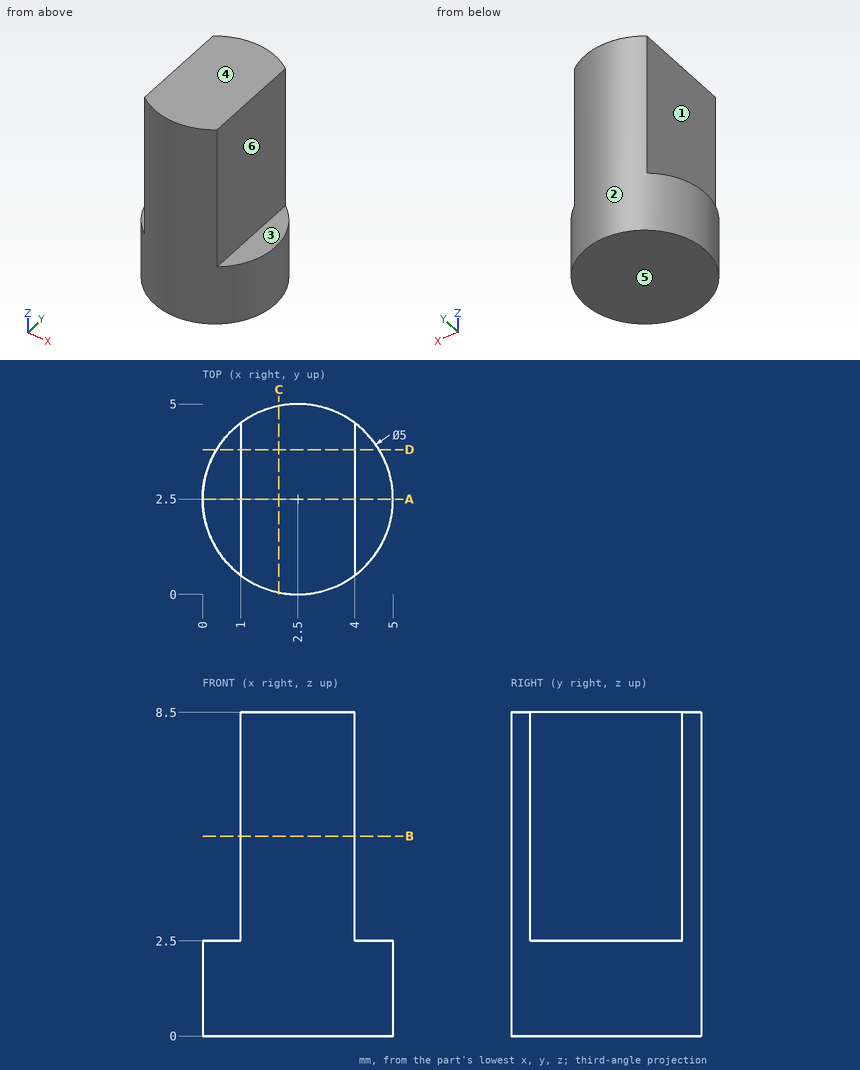
Geometry check sheet. Reference: drawing and pictorial views, mm from the part's lowest x, y, z. A direction names the side the tool comes from. Coordinates: 2 decimals unless noted, no trailing zeros. Write each loop counter-clockwise with the first axis right and the second up, starting at its lowest first coordinate (ties: lowest second). Pieces come first, ordered by that corner, then holes. Notation, with made-up numbers: (35, 60.25) - (92, 60.25) arc R25 ccw to (92, 76.25) - close; hole circle Ø3 at (-39, -15.75). An arc over 180 degrees is marked (long way). One line per question, with ' | ' between items. Start each with the question number.
1. Gauge pin test, flat ends, axial feed: P1, Ø1.5, axis at x = 3, z = 2, coming from the +Y side; P2, Ø1, axis at y = 0.5, z = 6, coming from the -X side; P3, Ø1.2, axis at y = 2.5, z = 5, coming from the +X side; P4, Ø0.5, axis at x = 0.5, y = 2.5, coming from the +Z side. Record the tip position at first contact, or that the pin passes through.
2. Material ranges on line 1 along Z through (x, y) = (4.1, 2.9); line 2 along Y through (x, z) = (1, 0.75); line 3 along X through (y, z) = (0.8, 7.5), recorded low to high.
3. Section check C-C (x = 2). Enter the section's corners in (y, z).
4. Access from +Z, -Z, +X, -X, +Y, -Y to the whole of each face (thin tool, end or side, straight path). Record for the marked faces 1, 2 and 3.
5. Section check A-A (y = 2.5). Enter the section's corners in (x, z).
6. Draft check along Z on the marked faces 4, 5 and 6. Enter one of: released by +Z, released by -Z, zero draft, split by the parting line, or undercut.
7. Section check D-D (y = 3.8). Enter the section's corners in (x, z).
8. Section check B-B (z = 5.25). Enter the section's corners in (x, y), plus the area to 3 significant figures.
Computed values:
1) P1: y = 5 | P2: x = 1 | P3: x = 4 | P4: z = 2.5
2) line 1: 0 to 2.5 | line 2: 0.5 to 4.5 | line 3: 1 to 4
3) outline: (0.05, 0) - (4.95, 0) - (4.95, 8.5) - (0.05, 8.5) - close
4) face 1: +Z, -X, +Y, -Y | face 2: +Z, -Z | face 3: +Z, +X, +Y, -Y
5) outline: (0, 0) - (5, 0) - (5, 2.5) - (4, 2.5) - (4, 8.5) - (1, 8.5) - (1, 2.5) - (0, 2.5) - close
6) face 4: released by +Z | face 5: released by -Z | face 6: zero draft
7) outline: (0.36, 0) - (4.64, 0) - (4.64, 2.5) - (4, 2.5) - (4, 8.5) - (1, 8.5) - (1, 2.5) - (0.36, 2.5) - close
8) outline: (1, 0.5) arc R2.5 ccw to (4, 0.5) - (4, 4.5) arc R2.5 ccw to (1, 4.5) - close | area: 14.0 mm²
